The model under review builds one solid part; all positions refer to its coordinate system, in mm. A direction names the side the tool comes from. Round coordinates to 2 decimals unless told otherwise and drop trailing zeros. Order: outer loops, then holes, each group sorted by start corner. A loop starts at its lowest first (then second) coordinate and runs counter-clockwise, first axis right, second up. Notation, with made-up numbers: M -35.75,66.25 L -28.75,66.25 A24 ccw -28.75,89.25 Z; hole C 88.25,12 d3. An arc over 180 degrees is marked long. Answer as a JSON object with one key per item and string values. Group by question number.
1. Machinability: for faces 1 (the face through (-20, -10, 23)), 2 (the face through (-2.237, -10.073, 15.919)), 3 (the face through (20.825, 8.427, 22.536)), 4 (the face through (-20, 10, 23)), which of the approach directions +Z, -Z, +X, -X, +Y, -Y give a long, thin tool a straight path to every point of the face, cutting with its end or side? Answer none if there is none.
2. Add section A-A on z = 29. State the section outline as (x, y) points (3 decimals), and give its area (3 significant figures).
3. Add section D-D on y = -8. State the section outline as (x, z) points (3 decimals).
4. Mouldability with a two-part tool opening along X and no side actions: class faces 5 (the face through (-1.38, 6.2, -3.13)), 6 (the face through (0, 0, 12.7)), 7 (the face through (-5, -5, 0)), 8 (the face through (-1.9, 10.4, 19.05)) as released by +X, released by -X, zero draft, split by the parting line, or undercut.
5. Add section B-B on y = 0. State the section outline as (x, z) points (3 decimals), and give its area (3 significant figures).
6. To check wall thickness, follow probe 1 along Y at (x, z) = (-0.5, 37) (3 decimals); probe 2 along Y at (x, z) = (0, 14.5) (3 decimals); probe 3 along Z at (x, y) = (9, 8.5). State the ranges of each line that lie inside material, in increasing order. Write a range as [from, to].
7. Clearance check with flat-ended pins moving along their axes: P1, Ø1.4, axis at x = -20.5, z = 12.5, coming from the +Y side; P2, Ø20.5, axis at x = 0, y = 0, coming from the +Z side; P3, Ø10, axis at x = 13.5, y = 16.5, coming from the -Z side. State where each tip first meets the part, or that it passes through.
```python
from build123d import *

# Parameters (mm, degrees)
F0_W      = 44.45
F0_H      = 44.45
F1_DEPTH  = 44.45
F2_R      = 10.31875
F3_DEPTH  = 31.75
F4_R      = 7.5
F5_DEPTH  = 50.8
F6_R      = 5.08
F8_DEPTH  = 50.8
F9_R      = 6.35
F10_DEPTH = 6.35
F11_R     = 12.7
F12_DEPTH = 25.4


with BuildPart() as f1:
    # F0 (on Top) → F1 (new body)
    with BuildSketch(Plane.XY):
        Rectangle(F0_W, F0_H)
    extrude(amount=F1_DEPTH)

    # F2 (on face) → F3 (cut)
    with BuildSketch(Plane.XY.offset(44.45)):
        Circle(F2_R)
    extrude(amount=-F3_DEPTH, mode=Mode.SUBTRACT)

    # F4 (on face) → F5 (cut)
    with BuildSketch(Plane.XY.offset(44.45)):
        with Locations((-17.5, 17.5)):
            Circle(F4_R)
        with Locations((17.5, 17.5)):
            Circle(F4_R)
        with Locations((17.5, -17.5)):
            Circle(F4_R)
        with Locations((-17.5, -17.5)):
            Circle(F4_R)
    extrude(amount=-F5_DEPTH, mode=Mode.SUBTRACT)

    # F6
    f6_edges = [f1.edges().sort_by_distance(p)[0] for p in [
        (-11.675537, -22.225, 22.225),
        (11.675537, -22.225, 22.225),
        (22.225, -11.675537, 22.225),
        (-11.675537, 22.225, 22.225),
        (11.675537, 22.225, 22.225),
        (22.225, 11.675537, 22.225),
    ]]
    fillet(f6_edges, radius=F6_R)

    # F7 (on face) → F8 (cut)
    with BuildSketch(Plane.XY.offset(44.45)):
        Polygon((-22.225, 10), (-17.5, 10), (-22.225, 11.6755365054), align=None)
        Polygon((-22.225, -12.5695262104), (-17.5, -10), (-22.225, -10), align=None)
    extrude(amount=-F8_DEPTH, mode=Mode.SUBTRACT)

    # F9 (on face) → F10 (join)
    with BuildSketch(Plane(origin=(0, 0, 0), x_dir=(1, 0, 0), z_dir=(0, 0, -1))):
        Circle(F9_R)
    extrude(amount=F10_DEPTH)

    # F11 (on face) → F12 (cut)
    with BuildSketch(Plane.XY.offset(44.45)):
        Circle(F11_R)
    extrude(amount=-F12_DEPTH, mode=Mode.SUBTRACT)


solid = f1.part
```
Recorded:
{
 "1": {"face 1": "+Z, -Z, -X, -Y", "face 2": "+Z", "face 3": "+Z, -Z, +X, +Y", "face 4": "+Z, -Z, -X, +Y"},
 "2": {"outline": "M -22.225,-10 L -17.5,-10 A7.5 cw -10.003,-17.288 A5.08 ccw -4.925,-22.225 L 4.925,-22.225 A5.08 ccw 10.003,-17.288 A7.5 cw 17.288,-10.003 A5.08 ccw 22.225,-4.925 L 22.225,4.925 A5.08 ccw 17.288,10.003 A7.5 cw 10.003,17.288 A5.08 ccw 4.925,22.225 L -4.925,22.225 A5.08 ccw -10.003,17.288 A7.5 cw -17.5,10 L -22.225,10 Z; hole C 0,0 d25.4", "area": "886 mm²"},
 "3": {"outline": "M -22.225,0 L 21.189,0 L 21.189,44.45 L 9.864,44.45 L 9.864,19.05 L 6.517,19.05 L 6.517,12.7 L -6.517,12.7 L -6.517,19.05 L -9.864,19.05 L -9.864,44.45 L -22.225,44.45 Z"},
 "4": {"face 5": "split by the parting line", "face 6": "undercut", "face 7": "zero draft", "face 8": "undercut"},
 "5": {"outline": "M -22.225,0 L -6.35,0 L -6.35,-6.35 L 6.35,-6.35 L 6.35,0 L 22.225,0 L 22.225,44.45 L 12.7,44.45 L 12.7,19.05 L 10.319,19.05 L 10.319,12.7 L -10.319,12.7 L -10.319,19.05 L -12.7,19.05 L -12.7,44.45 L -22.225,44.45 Z", "area": "1,280 mm²"},
 "6": {"probe 1": "y = [-22.225, -12.69], [12.69, 22.225]", "probe 2": "y = [-22.225, -10.319], [10.319, 22.225]", "probe 3": "z = [0, 19.05]"},
 "7": {"P1": "stops at y = 10", "P2": "stops at z = 12.7", "P3": "stops at z = 0"}
}
